Can you work these out from the model? Positions are in its coordinate system, mm. A direction names the side the tool comes from. Coordinates: 2 decimals unless noted, no trailing zeros. Order: outer loops, then holes, each group sorted by start corner. A loop starts at its lowest first (then second) coordinate and runs counter-clockwise, first axis right, second up. Notation, with made-up numbers: (31.5, 84) -> (36.5, 84) arc R20 ccw to (36.5, 94) -> close; hole circle Ø11 at (-33, 69). An arc over 180 degrees is marked (long way). Write item = value, one per line.
```python
from build123d import *

# Parameters (mm, degrees)
SKETCH1_R             = 39.007
SKETCH1_R_2           = 34.007
BOSS_EXTRUDE1_DEPTH   = 35
BOSS_EXTRUDE2_START   = 15
SKETCH2_R             = 5.007
BOSS_EXTRUDE2_DEPTH   = 5
BOSS_EXTRUDE2_2_DEPTH = 5
BOSS_EXTRUDE3_START   = -15
SKETCH3_R             = 5.007
BOSS_EXTRUDE3_DEPTH   = 5
BOSS_EXTRUDE3_2_DEPTH = 5
BOSS_EXTRUDE4_DEPTH   = 70
BOSS_EXTRUDE5_START   = -4
SKETCH5_R             = 3
BOSS_EXTRUDE5_DEPTH   = 4


with BuildPart() as part:
    # Sketch1 → Boss-Extrude1 (new, symmetric)
    with BuildSketch(Plane(origin=(0, 0, 0), x_dir=(0, 0, -1), z_dir=(1, 0, 0))):
        Circle(SKETCH1_R)
        Circle(SKETCH1_R_2, mode=Mode.SUBTRACT)
    extrude(amount=BOSS_EXTRUDE1_DEPTH, both=True)



with BuildPart() as body_2:
    # Sketch2 → Boss-Extrude2 (new body)
    with BuildSketch(Plane.XY.offset(BOSS_EXTRUDE2_START)):
        with BuildLine():
            Line((-35, -39.007), (35, -39.007))
            Line((35, -39.007), (25.596649495, -104.444761639))
            ThreePointArc((25.596649495, -104.444761639), (7.437713907, -121.532834549), (-13.266839867, -107.637848746))
            Line((-13.266839867, -107.637848746), (-35, -39.007))
        make_face()
        with Locations((5.8, -101.6)):
            Circle(SKETCH2_R, mode=Mode.SUBTRACT)
    extrude(amount=BOSS_EXTRUDE2_DEPTH)


with BuildPart() as body_3:
    # Sketch2 → Boss-Extrude2 2 (new body)
    with BuildSketch(Plane.XY.offset(BOSS_EXTRUDE2_START)):
        with BuildLine():
            Line((35, 39.007), (-35, 39.007))
            Line((-35, 39.007), (-13.266839867, 107.637848746))
            ThreePointArc((-13.266839867, 107.637848746), (7.437713907, 121.532834549), (25.596649495, 104.444761639))
            Line((25.596649495, 104.444761639), (35, 39.007))
        make_face()
        with Locations((5.8, 101.6)):
            Circle(SKETCH2_R, mode=Mode.SUBTRACT)
    extrude(amount=BOSS_EXTRUDE2_2_DEPTH)


with BuildPart() as body_4:
    # Sketch3 → Boss-Extrude3 (new body)
    with BuildSketch(Plane.XY.offset(BOSS_EXTRUDE3_START)):
        with BuildLine():
            Line((-35, -39.007), (-13.266839867, -107.637848746))
            ThreePointArc((-13.266839867, -107.637848746), (7.437713907, -121.532834549), (25.596649495, -104.444761639))
            Line((25.596649495, -104.444761639), (35, -39.007))
            Line((35, -39.007), (-35, -39.007))
        make_face()
        with Locations((5.8, -101.6)):
            Circle(SKETCH3_R, mode=Mode.SUBTRACT)
    extrude(amount=-BOSS_EXTRUDE3_DEPTH)


with BuildPart() as body_5:
    # Sketch3 → Boss-Extrude3 2 (new body)
    with BuildSketch(Plane.XY.offset(BOSS_EXTRUDE3_START)):
        with BuildLine():
            Line((-35, 39.007), (35, 39.007))
            Line((35, 39.007), (25.596649495, 104.444761639))
            ThreePointArc((25.596649495, 104.444761639), (7.437713907, 121.532834549), (-13.266839867, 107.637848746))
            Line((-13.266839867, 107.637848746), (-35, 39.007))
        make_face()
        with Locations((5.8, 101.6)):
            Circle(SKETCH3_R, mode=Mode.SUBTRACT)
    extrude(amount=-BOSS_EXTRUDE3_2_DEPTH)


with BuildPart() as part_1:
    add(part.part)

    add(body_2.part)  # Boss-Extrude4 merges body 2

    add(body_3.part)  # Boss-Extrude4 merges body 3

    add(body_4.part)  # Boss-Extrude4 merges body 4

    add(body_5.part)  # Boss-Extrude4 merges body 5
    # Sketch4 → Boss-Extrude4 (add)
    with BuildSketch(Plane(origin=(35, 0, 0), x_dir=(0, 0, -1), z_dir=(1, 0, 0))):
        with BuildLine():
            Line((20, -39.007), (15, -39.007))
            Line((15, -39.007), (15, -36.007583215))
            ThreePointArc((15, -36.007583215), (17.545232866, -34.838353186), (20, -33.489491621))
            Line((20, -33.489491621), (20, -39.007))
        make_face()
        with BuildLine():
            Line((-20, -39.007), (-15, -39.007))
            Line((-15, -39.007), (-15, -36.007583215))
            ThreePointArc((-15, -36.007583215), (-17.545232866, -34.838353186), (-20, -33.489491621))
            Line((-20, -33.489491621), (-20, -39.007))
        make_face()
        with BuildLine():
            Line((-20, 39.007), (-15, 39.007))
            Line((-15, 39.007), (-15, 36.007583215))
            ThreePointArc((-15, 36.007583215), (-17.545232866, 34.838353186), (-20, 33.489491621))
            Line((-20, 33.489491621), (-20, 39.007))
        make_face()
        with BuildLine():
            Line((20, 39.007), (15, 39.007))
            Line((15, 39.007), (15, 36.007583215))
            ThreePointArc((15, 36.007583215), (17.545232866, 34.838353186), (20, 33.489491621))
            Line((20, 33.489491621), (20, 39.007))
        make_face()
    extrude(amount=-BOSS_EXTRUDE4_DEPTH)

    # Sketch5 → Boss-Extrude5 (add)
    with BuildSketch(Plane.ZY.offset(25.9).offset(BOSS_EXTRUDE5_START)):
        with BuildLine():
            Line((50.098811723, 58.375353815), (20, 33.489491621))
            ThreePointArc((20, 33.489491621), (33.924077357, 19.253649641), (39.007, 0))
            Line((39.007, 0), (65.151054806, 45.703054903))
            ThreePointArc((65.151054806, 45.703054903), (62.911300808, 58.318387785), (50.098811723, 58.375353815))
        make_face()
        with Locations((56.470917013, 50.668455984)):
            Circle(SKETCH5_R, mode=Mode.SUBTRACT)
    extrude(amount=BOSS_EXTRUDE5_DEPTH)


solid = part_1.part
```
Item 1: I want a section at C-C, the plane z = 0. Please give me the cut outline in (x, y).
A:
outline = (-35, -39.01) -> (35, -39.01) -> (35, -34.01) -> (-35, -34.01) -> close; (-35, 34.01) -> (35, 34.01) -> (35, 39.01) -> (-35, 39.01) -> close
Item 2: For faces 4 (the flat face through (-23.872, 46.107, 35.26)), 5 (the flat face through (-25.9, 37, 43)), 6 (the flat face through (0, 67, -20)), which set-ups out of +Z, -Z, +X, -X, +Y, -Y let a thin tool reach every point of the face, with its end or its side?
A:
face_4 = +X, -X, +Y
face_5 = +Z, -X, +Y
face_6 = -Z, +X, -X, +Y
Item 3: I want a section at A-A, the plane x = 5.8. Give the number of separate pieces and of enclosed holes in the cut face, plus the area to 3 significant figures.
A:
separate_pieces = 5
enclosed_holes = 1
area = 2,680 mm2
Item 4: I'm going to push flat-ended pins straight in: P1, Ø3, axis at x = -3, z = -10, coming from the -Y side; P2, Ø3, axis at x = 10, z = 12, coming from the +Y side; P3, Ø2, axis at x = 11.5, y = -35, coming from the -Z side. Where does each tip first touch, or does it pass through?
A:
P1 = -38.07
P2 = 37.57
P3 = -20
Item 5: I want a section at B-B, the plane y = -55. Please give me the cut outline in (x, z).
A:
outline = (-29.94, -20) -> (32.7, -20) -> (32.7, -15) -> (-29.94, -15) -> close; (-29.94, 15) -> (32.7, 15) -> (32.7, 20) -> (-29.94, 20) -> close
Item 6: If we mould it in two halves opening along Y, with no side actions, what happens to faces 1 (the flat face through (-23.981, -73.803, 17.465)), 2 (the flat face through (-24.3, 72.8, 17.5)), 3 (the cylindrical face through (-23.872, 50.8, 53.474))? For each: pulls with the +Y half, pulls with the -Y half, needs draft (parallel to the pull), parting line crosses it, or undercut.
A:
face_1 = pulls with the -Y half
face_2 = pulls with the +Y half
face_3 = undercut
Item 7: If I drill on probe 1 along Z at (x, y) = (-11, -53); probe 2 along Y at (x, z) = (5.8, -18.5); probe 3 along Y at (x, z) = (-20, 0), over which ranges is the centre line in solid material (lowest first)?
A:
probe_1 = -20 to -15, 15 to 20
probe_2 = -121.6 to -106.61, -96.59 to -28.53, 28.53 to 96.59, 106.61 to 121.6
probe_3 = -39.01 to -34.01, 34.01 to 39.01
Item 8: I want a section at D-D, the plane y = -101.6. Please give me the cut outline in (x, z).
A:
outline = (-15.18, -20) -> (0.79, -20) -> (0.79, -15) -> (-15.18, -15) -> close; (-15.18, 15) -> (0.79, 15) -> (0.79, 20) -> (-15.18, 20) -> close; (10.81, -20) -> (26.01, -20) -> (26.01, -15) -> (10.81, -15) -> close; (10.81, 15) -> (26.01, 15) -> (26.01, 20) -> (10.81, 20) -> close
